from build123d import *

# Parameters (mm, degrees)
CROQUIS3_W              = 0.5
CROQUIS3_H              = 0.5
SALIENTE_EXTRUIR3_DEPTH = 25.4
CROQUIS4_W              = 0.912534335
CROQUIS4_H              = 5.586103973
CORTAR_EXTRUIR1_DEPTH   = 25.4
CORTAR_EXTRUIR2_REACH   = 946.999
CROQUIS5_W              = 0.5
CROQUIS5_H              = 1


with BuildPart() as part:
    # Croquis2 → Revolución1 (revolve)
    with BuildSketch(Plane(origin=(0, 0, 0), x_dir=(0, 0, -1), z_dir=(1, 0, 0))):
        with BuildLine():
            Line((0, -919.589259582), (2.95, -919.589259582))
            Line((2.95, -919.589259582), (2.95, -918.589259582))
            Line((2.95, -918.589259582), (2.5, -918.589259582))
            Line((2.5, -918.589259582), (2.5, -914.489259582))
            ThreePointArc((2.5, -914.489259582), (1.767766953, -912.721492629), (0, -911.989259582))
            Line((0, -911.989259582), (0, -919.589259582))
        make_face()
    revolve(axis=Axis((0, -1491.471633976, 0), (0, 1, 0)))

    # Croquis3 → Saliente-Extruir3 (add)
    with BuildSketch(Plane.XZ.offset(919.589259582)):
        with Locations((1.27, 0.018814001)):
            Rectangle(CROQUIS3_W, CROQUIS3_H)
        with Locations((-1.27, 0.018814001)):
            Rectangle(CROQUIS3_W, CROQUIS3_H)
    extrude(amount=SALIENTE_EXTRUIR3_DEPTH)

    # Croquis4 → Cortar-Extruir1 (cut)
    with BuildSketch(Plane(origin=(0, -918.589259582, 0), x_dir=(1, 0, 0), z_dir=(0, 1, 0))):
        with Locations((-2.956267168, 0.283432647)):
            Rectangle(CROQUIS4_W, CROQUIS4_H)
    extrude(amount=-CORTAR_EXTRUIR1_DEPTH, mode=Mode.SUBTRACT)

    # Croquis5 → Cortar-Extruir2 (cut, up to next)
    with BuildSketch(Plane.XY.offset(0.268814001), mode=Mode.PRIVATE) as cortar_extruir2_sk1:
        with Locations((-1.27, -944.489259582)):
            Rectangle(CROQUIS5_W, CROQUIS5_H)
    cortar_extruir2_tool1 = extrude(cortar_extruir2_sk1.sketch, amount=-CORTAR_EXTRUIR2_REACH, mode=Mode.PRIVATE) & part.part
    add(cortar_extruir2_tool1.solids().sort_by_distance((-1.27, -944.48926, 0.268814))[0], mode=Mode.SUBTRACT)


solid = part.part
CAD build for the part. Positions are in the model's coordinates, mm. A direction names the side the tool comes from. Round coordinates to 2 decimals unless told otherwise and drop trailing zeros. Loops run counter-clockwise (first coordinate to the right, second up) from the corner with the lowest first, then second, coordinate; pieces in that order, holes last. Notation, with made-up numbers: M 3.25,-25 L 19.25,-25 A31 cw 19.25,2 Z; hole C 77,48.5 d4. An arc over 180 degrees is marked long. One line per question, with ' | ' between items. Start each with the question number.
Item 1: Cut at A-A, the plane y = -925. Write the cut outline in (x, z), plus the area to 3 significant figures.
Item 2: Pin check, flat tips, straight feed: pin 1 Ø2 at (x, y) = (-1.5, -924.5) entering from +Z; pin 2 Ø0.6 at (y, z) = (-926.5, 0) entering from +X; pin 3 Ø1.5 at (x, z) = (1, -2) entering from +Y. Stop position of each tip, or through.
Item 3: Wall check: line 1 (X direction, y = -921, z = 0.1); line 2 (Z direction, x = -1.25, y = -942); line 3 (Y direction, x = 0.2, z = -2.55). Give the ranges that are in metal, low to high.
Item 4: Cut at C-C, the plane z = 2.05. Write the cut outline in (x, y), plus the area to 3 significant figures.
Item 5: Cut at B-B, the plane x = 0. Write the cut outline in (y, z).
Item 6: Which spindle directions (+Z, -Z, +X, -X, +Y, -Y) get a long thin tool onto all of the face, cutting with end or side? Do faces 1 (the cylindrical face through (2.44, -916.51, 0.54)), 2 (the cylindrical face through (2.948, -919.082, 0.107)). Say none if no direction does.
Responses:
1) outline: M -1.52,-0.23 L -1.02,-0.23 L -1.02,0.27 L -1.52,0.27 Z; M 1.02,-0.23 L 1.52,-0.23 L 1.52,0.27 L 1.02,0.27 Z | area: 0.500 mm²
2) pin 1: stops at z = 0.27 | pin 2: stops at x = 1.52 | pin 3: stops at y = -912.48
3) line 1: x = -1.52 to -1.02, 1.02 to 1.52 | line 2: z = -0.23 to 0.27 | line 3: y = -919.59 to -918.59
4) outline: M -2.12,-919.59 L 2.12,-919.59 L 2.12,-918.59 L 1.43,-918.59 L 1.43,-914.49 A1.43 ccw -1.43,-914.49 L -1.43,-918.59 L -2.12,-918.59 Z | area: 19.2 mm²
5) outline: M -919.59,-2.95 L -918.59,-2.95 L -918.59,-2.5 L -914.49,-2.5 A2.5 ccw -914.49,2.5 L -918.59,2.5 L -918.59,2.95 L -919.59,2.95 Z
6) face 1: +Y | face 2: +Y, -Y
